```python
from build123d import *

# Parameters (mm, degrees)
F0_R     = 32.1
F0_R_2   = 6.575
F3_DEPTH = 0.75
F4_DEPTH = 25
F1_R     = 11.575
F1_R_2   = 6.575
F5_DEPTH = 3
F6_SIZE  = 0.4


with BuildPart() as f3:
    # F0 (on Top) → F3 (new body)
    with BuildSketch(Plane.XY):
        Circle(F0_R)
        Circle(F0_R_2, mode=Mode.SUBTRACT)
    extrude(amount=F3_DEPTH)

    # F2 (on Top) → F4 (cut)
    with BuildSketch(Plane.XY):
        with BuildLine():
            ThreePointArc((11.5712747437, -0.2936423108), (11.5740686484, -0.1468329699), (11.575, 0))
            ThreePointArc((11.575, 0), (9.9500209897, 5.9141954063), (5.5313356711, 10.1678390376))
            ThreePointArc((5.5313356711, 10.1678390376), (0, 11.575), (-5.5313356711, 10.1678390376))
            ThreePointArc((-5.5313356711, 10.1678390376), (-10.0242440488, 5.7875), (-11.5712747437, -0.2936423108))
            ThreePointArc((-11.5712747437, -0.2936423108), (-10.0242440488, -5.7875), (-6.0399390726, -9.8741967268))
            ThreePointArc((-6.0399390726, -9.8741967268), (0, -11.575), (6.0399390726, -9.8741967268))
            ThreePointArc((6.0399390726, -9.8741967268), (10.0242440488, -5.7875), (11.5712747437, -0.2936423108))
        make_face()
        with BuildLine():
            ThreePointArc((-5.5313356711, 10.1678390376), (0, 11.575), (5.5313356711, 10.1678390376))
            ThreePointArc((5.5313356711, 10.1678390376), (7.2175038611, 9.9127061865), (8.6749690104, 10.7981728857))
            ThreePointArc((8.6749690104, 10.7981728857), (9.1772189992, 12.8554118424), (7.9206815333, 14.5599941294))
            ThreePointArc((7.9206815333, 14.5599941294), (0, 16.575), (-7.9206815333, 14.5599941294))
            ThreePointArc((-7.9206815333, 14.5599941294), (-9.1772189992, 12.8554118424), (-8.6749690104, 10.7981728857))
            ThreePointArc((-8.6749690104, 10.7981728857), (-7.2175038611, 9.9127061865), (-5.5313356711, 10.1678390376))
        make_face()
        with BuildLine():
            ThreePointArc((13.6889765386, 2.1136570972), (12.1934073083, 1.2941886024), (11.5712747437, -0.2936423108))
            ThreePointArc((11.5712747437, -0.2936423108), (10.0242440488, -5.7875), (6.0399390726, -9.8741967268))
            ThreePointArc((6.0399390726, -9.8741967268), (4.9759034472, -11.2068947889), (5.0140075282, -12.9118299829))
            ThreePointArc((5.0140075282, -12.9118299829), (6.544503732, -14.3754107106), (8.6489840283, -14.1395084878))
            ThreePointArc((8.6489840283, -14.1395084878), (14.3543710677, -8.2875), (16.5696655617, -0.4204856416))
            ThreePointArc((16.5696655617, -0.4204856416), (15.7217227312, 1.5199988682), (13.6889765386, 2.1136570972))
        make_face()
        with BuildLine():
            ThreePointArc((-6.0399390726, -9.8741967268), (-10.0242440488, -5.7875), (-11.5712747437, -0.2936423108))
            ThreePointArc((-11.5712747437, -0.2936423108), (-12.1934073083, 1.2941886024), (-13.6889765386, 2.1136570972))
            ThreePointArc((-13.6889765386, 2.1136570972), (-15.7217227312, 1.5199988682), (-16.5696655617, -0.4204856416))
            ThreePointArc((-16.5696655617, -0.4204856416), (-14.3543710677, -8.2875), (-8.6489840283, -14.1395084878))
            ThreePointArc((-8.6489840283, -14.1395084878), (-6.544503732, -14.3754107106), (-5.0140075282, -12.9118299829))
            ThreePointArc((-5.0140075282, -12.9118299829), (-4.9759034472, -11.2068947889), (-6.0399390726, -9.8741967268))
        make_face()
    extrude(amount=F4_DEPTH, mode=Mode.SUBTRACT)

    # F1 (on Top) → F5 (join)
    with BuildSketch(Plane.XY):
        Circle(F1_R)
        Circle(F1_R_2, mode=Mode.SUBTRACT)
    extrude(amount=F5_DEPTH)

    # F6
    f6_edges = [f3.edges().sort_by_distance(p)[0] for p in [
        (-32.1, 0, 0),
        (8.922086, 11.169244, 0),
        (0, 11.575, 0),
        (-8.922086, 11.169244, 0),
        (0, 16.575, 0),
        (-14.133892, 2.142131, 0),
        (-10.024244, -5.7875, 0),
        (-5.211806, -13.311375, 0),
        (-14.354371, -8.2875, 0),
        (5.211806, -13.311375, 0),
        (10.024244, -5.7875, 0),
        (14.133892, 2.142131, 0),
        (14.354371, -8.2875, 0),
        (-6.575, 0, 0),
    ]]
    chamfer(f6_edges, length=F6_SIZE)


solid = f3.part
```
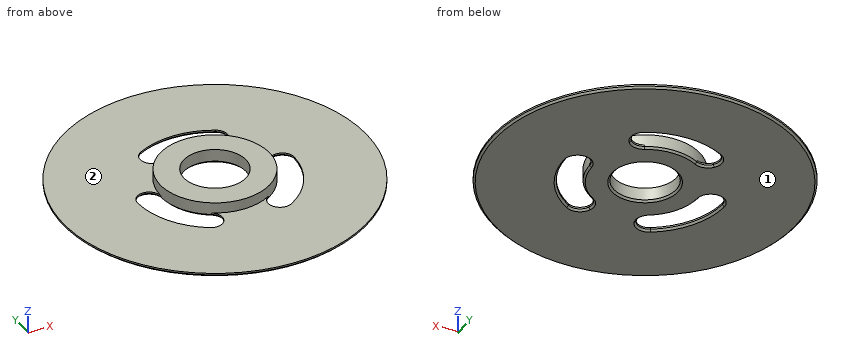
The listing builds one solid part. Answer for the finished solid, in the listing's coordinates (mm). Face numbers are marked on the shaded views. A direction names the side the tool comes from. Coordinates: 2 decimals unless noted, no trailing zeros. Write each loop counter-clockwise with the first axis right and the second up, starting at its lowest first coordinate (ties: lowest second). Pieces come first, ordered by that corner, then holes. Notation, with made-up numbers: M 75.25,82 L 105.25,82 A19 ccw 105.25,97 Z; hole C 48.25,60 d7. An arc over 180 degrees is marked long. Use a Markdown table: item, result. Add a question column.
1. Given P1, Ø8, axis at x = 19, y = -2.5, coming from the +Z side, flat-ended and moving along its own axis, determine where the tip first touches the part or whether it passes through.
2. Straight lines are drawn through the part: line 1 along Y through (x, z) = (0, 1.95) (3 decimals); line 2 along Y through (x, z) = (-3, 1.6); line 3 along Z through (x, y) = (-1.5, -25). For each, find the intervals that lie inside material, in ascending order. Write a range as [from, to].
3. Section B-B (z = 2.5) is taken. Give the vertices of the cut face in (x, y) (3 decimals), plus the area to 3 significant figures.
4. Section A-A (x = 0) is taken. Give the vertices of the cut face in (y, z) (3 decimals).
5. Which of the six approach directions +Z, -Z, +X, -X, +Y, -Y give full straight-line access (tool end or side, diameter ignored) to the marked faces 1 and 2?
Data:
| question | item | result |
|---|---|---|
| 1 | P1 | stops at z = 0.75 |
| 2 | line 1 | y = [-11.575, -6.575], [6.575, 11.575] |
| 2 | line 2 | y = [-11.18, -5.85], [5.85, 11.18] |
| 2 | line 3 | z = [0, 0.75] |
| 3 | outline | C 0,0 d23.15; hole C 0,0 d13.15 |
| 3 | area | 285 mm2 |
| 4 | outline | M -32.1,0.4 L -31.7,0 L -6.975,0 L -6.575,0.4 L -6.575,3 L -11.575,3 L -11.575,0.75 L -32.1,0.75 Z; M 6.575,0.4 L 6.975,0 L 11.175,0 L 11.575,0.4 L 11.575,3 L 6.575,3 Z; M 16.575,0.4 L 16.975,0 L 31.7,0 L 32.1,0.4 L 32.1,0.75 L 16.575,0.75 Z |
| 5 | face 1 | -Z, +X, -X, +Y, -Y |
| 5 | face 2 | +Z |
